For this review, use the dimensioned drawing (mm, ordinates from the lowest corner) and the shaded views. A direction names the side the tool comes from. Coordinates: 2 decimals unless noted, no trailing zeros. Order: outer loops, then holes, each group sorted by start corner. A loop starts at its lowest first (then second) coordinate and runs counter-clockwise, first axis right, second up. Notation, with made-up numbers: M -7,-22 L 48,-22 A28 cw 48,5 Z; hole C 5.25,32 d5. An arc over 180 degrees is marked long. Answer in a Markdown table with one row per item.
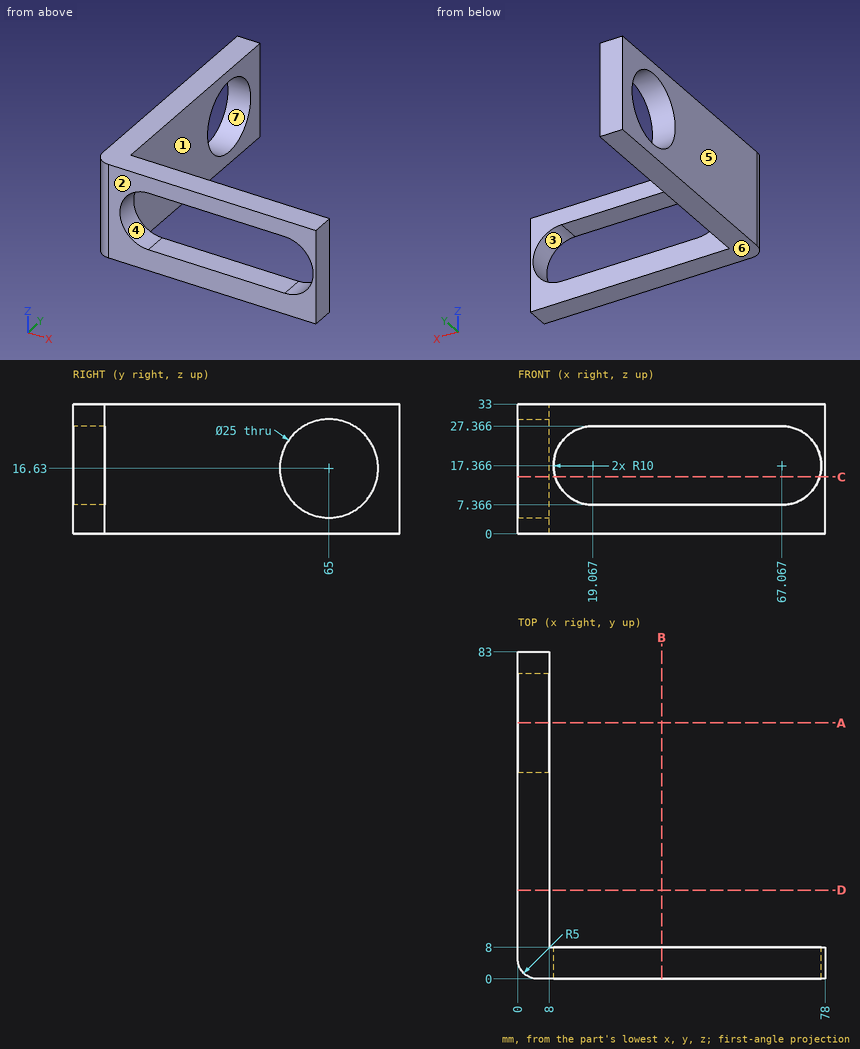
(1) To check wall thickness, follow line 1 (Z direction, x = 3, y = 65); line 2 (Y direction, x = 63, z = 28.5). State the ranges of each line that lie inside material, in increasing order. Write a range as [from, to].
Report:
| item | result |
|---|---|
| line 1 | [0, 4.13], [29.13, 33] |
| line 2 | [0, 8] |
(2) The part is to be moulded in two halves that separate along Z. For the marked faces 4, 5, 6 and 7, say which applies: +Z half, -Z half, draft (parallel to the pull), parting line (faces both ways), or undercut.
Report:
| item | result |
|---|---|
| face 4 | undercut |
| face 5 | draft |
| face 6 | -Z half |
| face 7 | undercut |
(3) Take a section at D-D (y = 22.5). Write out the cut boundary in (x, z).
Report:
| item | result |
|---|---|
| outline | M 0,0 L 8,0 L 8,33 L 0,33 Z |
(4) Machinability: for the marked faces 1, 2 and 3, which of the approach directions +Z, -Z, +X, -X, +Y, -Y give a long, thin tool a straight path to every point of the face, cutting with its end or side? Answer none if there is none.
Report:
| item | result |
|---|---|
| face 1 | +Z, -Z, +X, +Y |
| face 2 | +Z, -Z, +X, -X, -Y |
| face 3 | +Y, -Y |
(5) Take a section at B-B (x = 36.5). Write out the cut boundary in (y, z).
Report:
| item | result |
|---|---|
| outline | M 0,0 L 8,0 L 8,7.37 L 0,7.37 Z; M 0,27.37 L 8,27.37 L 8,33 L 0,33 Z |
(6) Take a section at C-C (z = 14.5). Write out the cut boundary in (x, y), then the cut area to 3 significant figures.
Report:
| item | result |
|---|---|
| outline | M 0,5 A5 ccw 5,0 L 9.49,0 L 9.49,8 L 8,8 L 8,52.68 L 0,52.68 Z; M 0,77.32 L 8,77.32 L 8,83 L 0,83 Z; M 76.65,0 L 78,0 L 78,8 L 76.65,8 Z |
| area | 484 mm^2 |
(7) Insertion check: P1, Ø10, axis at x = 57.5, z = 6.5, coming from the +Y side; P2, Ø6, axis at y = 57, z = 27.5, coming from the +X side; P3, Ø4, axis at x = 34.5, y = 2.5, coming from the -Z side. Each pin has a flat end and moves straight along its axis. Give the tip position at first contact, or say it passes through.
Report:
| item | result |
|---|---|
| P1 | y = 8 |
| P2 | x = 8 |
| P3 | z = 0 |
(8) Take a section at A-A (y = 65). Write out the cut boundary in (x, z).
Report:
| item | result |
|---|---|
| outline | M 0,0 L 8,0 L 8,4.13 L 0,4.13 Z; M 0,29.13 L 8,29.13 L 8,33 L 0,33 Z |
